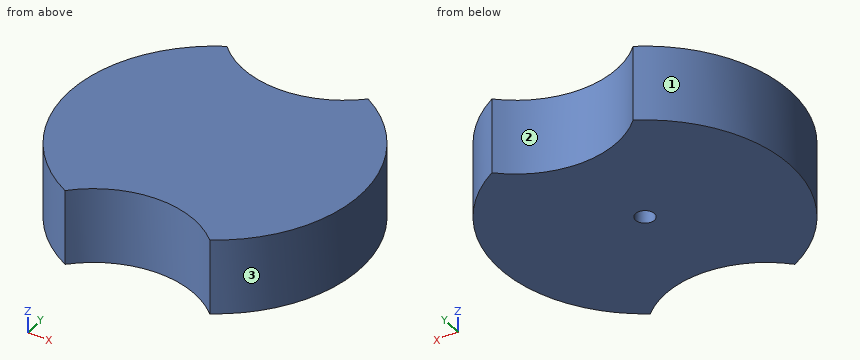
from build123d import *

# Parameters (mm, degrees)
SKETCH_1_R          = 38.5
EXTRUDE_2_DEPTH     = 20
CUT_EXTRUDE_1_DEPTH = 20
SKETCH_4_R          = 2.5
CUT_EXTRUDE_2_DEPTH = 8


with BuildPart() as part:
    # Эскиз1 → Бобышка-Вытянуть2 (new body)
    with BuildSketch(Plane.XY):
        Circle(SKETCH_1_R)
    extrude(amount=EXTRUDE_2_DEPTH)

    # Эскиз3 → Вырез-Вытянуть1 (cut)
    with BuildSketch(Plane.XY):
        with BuildLine():
            ThreePointArc((-18.301346902, 33.871975165), (0.496314005, 25.656261649), (19.597654242, 33.138828407))
            ThreePointArc((19.597654242, 33.138828407), (0.744633616, 38.492798298), (-18.301346902, 33.871975165))
        make_face()
        with BuildLine():
            ThreePointArc((-18.301346902, -33.871975165), (0.496314005, -25.656261649), (19.597654242, -33.138828407))
            ThreePointArc((19.597654242, -33.138828407), (0.744633616, -38.492798298), (-18.301346902, -33.871975165))
        make_face()
    extrude(amount=CUT_EXTRUDE_1_DEPTH, mode=Mode.SUBTRACT)

    # Эскиз4 → Вырез-Вытянуть2 (cut)
    with BuildSketch(Plane.XY):
        Circle(SKETCH_4_R)
    extrude(amount=CUT_EXTRUDE_2_DEPTH, mode=Mode.SUBTRACT)


solid = part.part
Geometry: final body of the model. Coordinates: model frame, mm. Face numbers are marked on the shaded views. Coordinates: 2 decimals unless noted, no trailing zeros. Order: outer loops, then holes, each group sorted by start corner. A loop starts at its lowest first (then second) coordinate and runs counter-clockwise, first axis right, second up.
1) First-contact query: P1, Ø12, axis at y = 27, z = 16, coming from the -X side; P2, Ø1, axis at y = 8, z = 13.5, coming from the +X side; P3, Ø8, axis at x = -1, z = 2, coming from the +Y side. Flat tips, straight axial feed; report the tip coordinate or a pass-through.
Result sheet:
P1: stops at x = -32.27
P2: stops at x = 37.76
P3: stops at y = 26.33
2) Draft query along X for the marked faces 1, 2 and 3. Return one class per face: released by +X, released by -X, zero draft, split by the parting line, or undercut.
Result sheet:
face 1: released by -X
face 2: undercut
face 3: released by +X
3) Section D-D (z = 18.5). Return loops of the section in (x, y).
Result sheet:
outline: (-18.3, -33.87) arc R26.8 cw to (19.6, -33.14) arc R38.5 ccw to (19.6, 33.14) arc R26.8 cw to (-18.3, 33.87) arc R38.5 ccw to start
4) Section B-B (y = 0). Return loops of the section in (x, z).
Result sheet:
outline: (-38.5, 0) - (-2.5, 0) - (-2.5, 8) - (2.5, 8) - (2.5, 0) - (38.5, 0) - (38.5, 20) - (-38.5, 20) - close
5) Section C-C (x = 0). Return loops of the section in (y, z), then the cut area to 3 significant figures.
Result sheet:
outline: (-25.67, 0) - (-2.5, 0) - (-2.5, 8) - (2.5, 8) - (2.5, 0) - (25.67, 0) - (25.67, 20) - (-25.67, 20) - close
area: 987 mm2
6) Ray query, probe 1 along Y at (x, z) = (0, 2.75); probe 2 along X at (y, z) = (-28, 8.75); probe 3 along Y at (x, z) = (-20.5, 6.75). Return the intervals inside material, ascending.
Result sheet:
probe 1: y = -25.67 to -2.5, 2.5 to 25.67
probe 2: x = -26.42 to -9.96, 11.99 to 26.42
probe 3: y = -32.59 to 32.59
7) Section A-A (z = 5.25). Return loops of the section in (x, y), then the cut area to 3 significant figures.
Result sheet:
outline: (-18.3, -33.87) arc R26.8 cw to (19.6, -33.14) arc R38.5 ccw to (19.6, 33.14) arc R26.8 cw to (-18.3, 33.87) arc R38.5 ccw to start; hole circle Ø5 at (0, 0)
area: 3,970 mm2
